Design review of the part built by this model. Coordinates are the model's own, in mm. Face numbers are marked on the shaded views. A direction names the side the tool comes from. Give positions to 0.01 mm unless a question says otherwise; leave off trailing zeros. Loops run counter-clockwise (first coordinate to the right, second up) from the corner with the lowest first, then second, coordinate; pieces in that order, holes last. Notation, with made-up numbers: (63.25, 85.25) -> (95.25, 85.25) arc R25 ccw to (95.25, 116.25) -> close; hole circle Ø7 at (-18, -12.75). An arc over 180 degrees is marked (long way). Use CSV: the item, a comma, the result in double quotes. Start each with the question number.
Item 1: We need section A-A (y = 0). State the section outline as (x, z) points, plus the area to 3 significant figures.
Item 2: The part is to be moulded in two halves that separate along X. For the marked faces 3, 4 and 5, say which applies: +X half, -X half, draft (parallel to the pull), parting line (faces both ways), or undercut.
Item 3: Clearance check with flat-ended pins moving along their axes: pin 1 (5.5 mm diameter, centred on y = -27, z = 8, fed in from +X); pin 2 (8 mm diameter, centred on y = -25, z = 11, fed in from -X); pin 3 (1.5 mm diameter, centred on x = -0.5, z = 14.5, fed in from -Y). State where each tip first meets the part, or that it passes through.
Item 4: Wall thickness on line 1 along Z through (x, y) = (0, -27); line 2 along X through (y, z) = (0, 9.25); line 3 along X through (y, z) = (-18.5, 8.5): over which ranges is each line inside the solid? List them lowest first. Write a range as from..to.
Item 5: We need section D-D (z = 11). State the section outline as (x, y) points, plus the area to 3 significant figures.
Item 6: We need section B-B (z = 8.5). State the section outline as (x, y) points, plus the area to 3 significant figures.
Item 7: For the marked faces 1 and 2, list the 3-axis set-ups (+Z, -Z, +X, -X, +Y, -Y) from which the entire face can be reached by the end or side of a thin tool; tool diameter is ignored.
from build123d import *

# Parameters (mm, degrees)
F0_R     = 8
F1_DEPTH = 16
F3_DEPTH = 25
F4_R     = 1.5
F5_R     = 7.99999
F6_R     = 10
F7_R     = 2.1
F8_DEPTH = 25


# Not quite as in the source:
# - a fillet or chamfer is up to 0.001 mm smaller than in the source, because OpenCascade refuses the exact size


with BuildPart() as f1:
    # F0 (on Top) → F1 (new body)
    with BuildSketch(Plane.XY):
        with BuildLine():
            Line((2.5, -35), (2.5, -10.7121426428))
            ThreePointArc((2.5, -10.7121426428), (0, 11), (-2.5, -10.7121426428))
            Line((-2.5, -10.7121426428), (-2.5, -35))
            Line((-2.5, -35), (2.5, -35))
        make_face()
        Circle(F0_R, mode=Mode.SUBTRACT)
    extrude(amount=F1_DEPTH)

    # F2 (on face) → F3 (cut)
    with BuildSketch(Plane.XY.offset(16)):
        with BuildLine():
            ThreePointArc((-7, 3.8729833462), (0, 8), (7, 3.8729833462))
            Line((7, 3.8729833462), (7, 8.4852813742))
            ThreePointArc((7, 8.4852813742), (0, 11), (-7, 8.4852813742))
            Line((-7, 8.4852813742), (-7, 3.8729833462))
        make_face()
    extrude(amount=-F3_DEPTH, mode=Mode.SUBTRACT)

    # F4
    f4_edges = [f1.edges().sort_by_distance(p)[0] for p in [
        (-7, 8.485281, 8),
        (7, 8.485281, 8),
    ]]
    fillet(f4_edges, radius=F4_R)

    # F5 (radius 8 in the source; OpenCascade refuses exactly that, so slightly less here)
    f5_edges = [f1.edges().sort_by_distance(p)[0] for p in [
        (0, -35, 16),
        (0, -35, 0),
    ]]
    fillet(f5_edges, radius=F5_R)

    # F6
    f6_edges = [f1.edges().sort_by_distance(p)[0] for p in [
        (-2.5, -10.712143, 8),
        (2.5, -10.712143, 8),
    ]]
    fillet(f6_edges, radius=F6_R)

    # F7 (on face) → F8 (cut)
    with BuildSketch(Plane(origin=(-2.5, 0, 0), x_dir=(0, -1, 0), z_dir=(-1, 0, 0))):
        with Locations((27, 8)):
            Circle(F7_R)
    extrude(amount=-F8_DEPTH, mode=Mode.SUBTRACT)


solid = f1.part
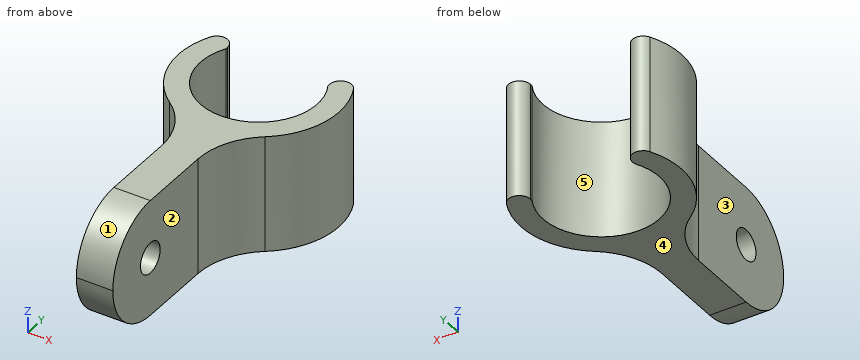
Results found:
1,outline,"(-11, 0) -> (-8, 0) -> (-8, 16) -> (-11, 16) -> close; (8, 0) -> (11, 0) -> (11, 16) -> (8, 16) -> close"
1,area,"96.0 mm²"
2,face 3,"-X half"
2,face 4,"draft"
2,face 5,"undercut"
3,pin 1,"x = 2.5"
3,pin 2,"x = -2.5"
3,pin 3,"y = -32.56"
4,line 1,"0..5.9, 10.1..16"
4,line 2,"-11..-8, 8..11"
4,line 3,"-2.5..2.5"
5,outline,"(-9.84, 4.91) arc R11 ccw to (-6.55, -8.84) arc R10 cw to (-2.5, -16.87) -> (-2.5, -34.42) -> (2.5, -34.42) -> (2.5, -16.87) arc R10 cw to (6.55, -8.84) arc R11 ccw to (9.84, 4.91) arc R1.5 ccw to (7, 4.24) -> (7, 3.87) arc R8 cw (long way) to (-7, 3.87) -> (-7, 4.24) arc R1.5 ccw to start"
5,area,"251 mm²"
6,outline,"(-9.84, 4.91) arc R11 ccw to (-6.55, -8.84) arc R10 cw to (-2.5, -16.87) -> (-2.5, -24.96) -> (2.5, -24.96) -> (2.5, -16.87) arc R10 cw to (6.55, -8.84) arc R11 ccw to (9.84, 4.91) arc R1.5 ccw to (7, 4.24) -> (7, 3.87) arc R8 cw (long way) to (-7, 3.87) -> (-7, 4.24) arc R1.5 ccw to start; (-2.5, -34.98) -> (2.5, -34.98) -> (2.5, -29.04) -> (-2.5, -29.04) -> close"
6,area,"234 mm²"
7,face 1,"+Z, +X, -X, -Y"
7,face 2,"+Z, -Z, +X, -Y"
